For this review, take the finished solid that the model builds, in its own axes (mm). A direction names the side the tool comes from. Give positions to 0.01 mm unless a question says otherwise; leave off trailing zeros. Write each loop counter-clockwise with the first axis right and the second up, starting at its lowest first coordinate (ties: lowest second). Pieces come first, ordered by that corner, then holes. Notation, with made-up numbers: M 22,65.5 L 67,65.5 A20 cw 67,84.5 Z; hole C 19.5,37.25 d8. An arc over 180 degrees is marked long. Write item = value, one per line.
```python
from build123d import *

# Parameters (mm, degrees)
SKETCH_1_R          = 1.5
SKETCH_1_R_2        = 2.5
EXTRUDE_1_DEPTH     = 10.3
CUT_EXTRUDE_1_DEPTH = 3.8
FILLET_1_R          = 2
FILLET_2_R          = 1
FILLET_3_R          = 1
FILLET_4_R          = 1


with BuildPart() as part:
    # 草图1 → 凸台-拉伸1 (new body)
    with BuildSketch(Plane(origin=(0, 0, 0), x_dir=(1, 0, 0), z_dir=(0, 1, 0))):
        Polygon((0, 12), (0, 0), (12, 0), (12, 0.9), (18, 0.9), (18, 0), (30, 0), (30, 12), (18, 12), (18, 11.1), (12, 11.1), (12, 12), align=None)
        with Locations(Location((2.5, 3, 0), (0, 0, 90))):
            Circle(SKETCH_1_R, mode=Mode.SUBTRACT)
        with Locations(Location((15, 6, 0), (0, 0, 90))):
            Circle(SKETCH_1_R_2, mode=Mode.SUBTRACT)
        with Locations(Location((27.5, 3, 0), (0, 0, 90))):
            Circle(SKETCH_1_R, mode=Mode.SUBTRACT)
        with Locations(Location((2.5, 9, 0), (0, 0, 90))):
            Circle(SKETCH_1_R, mode=Mode.SUBTRACT)
        with Locations(Location((27.5, 9, 0), (0, 0, 90))):
            Circle(SKETCH_1_R, mode=Mode.SUBTRACT)
    extrude(amount=EXTRUDE_1_DEPTH)

    # 草图2 → 切除-拉伸1 (cut)
    with BuildSketch(Plane(origin=(0, 10.3, 0), x_dir=(1, 0, 0), z_dir=(0, 1, 0))):
        Polygon((10.265727793, 6), (12.632863896, 1.9), (17.367136104, 1.9), (19.734272207, 6), (17.367136104, 10.1), (12.632863896, 10.1), align=None)
    extrude(amount=-CUT_EXTRUDE_1_DEPTH, mode=Mode.SUBTRACT)

    # 圆角1
    fillet_1_edges = [part.edges().sort_by_distance(p)[0] for p in [
        (30, 5.15, -12),
        (30, 5.15, 0),
        (0, 5.15, 0),
        (0, 5.15, -12),
    ]]
    fillet(fillet_1_edges, radius=FILLET_1_R)

    # 圆角2
    fillet_2_edges = [part.edges().sort_by_distance(p)[0] for p in [
        (10.265727793, 8.4, -6),
        (12.632863896, 8.4, -10.1),
        (17.367136104, 8.4, -10.1),
        (19.734272207, 8.4, -6),
        (17.367136104, 8.4, -1.9),
        (12.632863896, 8.4, -1.9),
    ]]
    fillet(fillet_2_edges, radius=FILLET_2_R)

    # 圆角3
    # the kernel refuses this fillet: 1 mm, written as the material it adds along each edge
    with BuildSketch(Plane(origin=(12, 0, -0.9), x_dir=(0, 0, 1), z_dir=(0, 1, 0))) as fillet_3_piece_1:
        with BuildLine():
            CenterArc((1, 0.994987437), FILLET_3_R, 180, 84.260829523)
            Line((0, 0.994987437), (-0.02, 0.994987437))
            Line((-0.02, 0.994987437), (-0.02, 0))
            Line((-0.02, 0), (0, -0.02))
            ThreePointArc((0, -0.02), (0.45, -0.02), (0.898, -0.019899749))
            Line((0.898, -0.019899749), (0.9, 0))
        make_face()
    extrude(amount=10.3)
    with BuildSketch(Plane(origin=(18, 0, -0.9), x_dir=(-1, 0, 0), z_dir=(0, 1, 0))) as fillet_3_piece_2:
        with BuildLine():
            CenterArc((0.994987437, 1), FILLET_3_R, 185.739170477, 84.260829523)
            Line((0, 0.9), (-0.019899749, 0.898))
            ThreePointArc((-0.019899749, 0.898), (-0.02, 0.45), (-0.02, 0))
            Line((-0.02, 0), (0, -0.02))
            Line((0, -0.02), (0.994987437, -0.02))
            Line((0.994987437, -0.02), (0.994987437, 0))
        make_face()
    extrude(amount=10.3)
    with BuildSketch(Plane(origin=(12, 0, -11.1), x_dir=(0, 0, -1), z_dir=(0, 1, 0))) as fillet_3_piece_3:
        with BuildLine():
            CenterArc((1, -0.994987437), FILLET_3_R, 95.739170477, 84.260829523)
            Line((0, -0.994987437), (-0.02, -0.994987437))
            Line((-0.02, -0.994987437), (-0.02, 0))
            Line((-0.02, 0), (0, 0.02))
            ThreePointArc((0, 0.02), (0.45, 0.02), (0.898, 0.019899749))
            Line((0.898, 0.019899749), (0.9, 0))
        make_face()
    extrude(amount=10.3)
    with BuildSketch(Plane(origin=(18, 0, -11.1), x_dir=(-1, 0, 0), z_dir=(0, 1, 0))) as fillet_3_piece_4:
        with BuildLine():
            CenterArc((0.994987437, -1), FILLET_3_R, 90, 84.260829523)
            Line((0, -0.9), (-0.019899749, -0.898))
            ThreePointArc((-0.019899749, -0.898), (-0.02, -0.45), (-0.02, 0))
            Line((-0.02, 0), (0, 0.02))
            Line((0, 0.02), (0.994987437, 0.02))
            Line((0.994987437, 0.02), (0.994987437, 0))
        make_face()
    extrude(amount=10.3)

    # 圆角4
    fillet_4_edges = [part.edges().sort_by_distance(p)[0] for p in [
        (18, 5.15, 0),
        (12, 5.15, 0),
        (12, 5.15, -12),
        (18, 5.15, -12),
    ]]
    fillet(fillet_4_edges, radius=FILLET_4_R)


solid = part.part
```
1. Machinability: for faces 4 (the face through (26, 5, -9)), 5 (the face through (15, 5, -11.1)), 6 (the face through (18.56, 8.43, -8.03)), which of the approach directions +Z, -Z, +X, -X, +Y, -Y give a long, thin tool a straight path to every point of the face, cutting with its end or side? Answer none if there is none.
Responses:
face_4 = +Y, -Y
face_5 = -Z, +Y, -Y
face_6 = +Y
2. We need section A-A, the plane z = -6. Write out the cut boundary in (x, y).
Responses:
outline = M 0,0 L 12.5,0 L 12.5,6.5 L 10.42,6.5 L 10.42,10.3 L 0,10.3 Z; M 17.5,0 L 30,0 L 30,10.3 L 19.58,10.3 L 19.58,6.5 L 17.5,6.5 Z
3. We need section C-C, the plane x = 15. Write out the cut boundary in (y, z), then the cut area to 3 significant figures.
Responses:
outline = M 0,-11.1 L 10.3,-11.1 L 10.3,-10.1 L 6.5,-10.1 L 6.5,-8.5 L 0,-8.5 Z; M 0,-3.5 L 6.5,-3.5 L 6.5,-1.9 L 10.3,-1.9 L 10.3,-0.9 L 0,-0.9 Z
area = 41.4 mm2
4. We need section B-B, the plane x = 2.5. Write out the cut boundary in (y, z), then the cut area to 3 significant figures.
Responses:
outline = M 0,-12 L 10.3,-12 L 10.3,-10.5 L 0,-10.5 Z; M 0,-7.5 L 10.3,-7.5 L 10.3,-4.5 L 0,-4.5 Z; M 0,-1.5 L 10.3,-1.5 L 10.3,0 L 0,0 Z
area = 61.8 mm2
5. For line 1 along X through (y, z) = (6, -9); line 2 along Z through (x, y) = (27.5, 5); line 3 along X through (y, z) = (8.25, -3), list the stretches that pass through material, from the lowest coordinate up. Write a range as from..to.
Responses:
line_1 = 0..1, 4..26, 29..30
line_2 = -12..-10.5, -7.5..-4.5, -1.5..0
line_3 = 0..1, 4..12, 18..26, 29..30
6. We need section D-D, the plane y = 1.25. Write out the cut boundary in (x, z), then the cut area to 3 significant figures.
Responses:
outline = M 0,-10 A2 ccw 2,-12 L 11.32,-12 A1 ccw 12.16,-11.55 A1 cw 12.99,-11.1 L 17.01,-11.1 A1 cw 17.84,-11.55 A1 ccw 18.68,-12 L 28,-12 A2 ccw 30,-10 L 30,-2 A2 ccw 28,0 L 18.68,0 A1 ccw 17.84,-0.45 A1 cw 17.01,-0.9 L 12.99,-0.9 A1 cw 12.16,-0.45 A1 ccw 11.32,0 L 2,0 A2 ccw 0,-2 Z; hole C 2.5,-9 d3; hole C 2.5,-3 d3; hole C 15,-6 d5; hole C 27.5,-9 d3; hole C 27.5,-3 d3
area = 298 mm2
7. The part is to be moulded in two halves that separate along X. For faces 1 (the face through (15, 5, -0.9)), 2 (the face through (0.57, 5.22, -11.4)), 3 (the face through (23, 5, -12)), say which applies: +X half, -X half, draft (parallel to the pull), parting line (faces both ways), or undercut.
Responses:
face_1 = undercut
face_2 = -X half
face_3 = draft
8. Insertion check: P1, Ø6, axis at x = 15, z = -6, coming from the -Y side; P2, Ø1.2, axis at x = 16, y = 7.5, coming from the +Z side; P3, Ø1.1, axis at x = 15, y = 8.5, coming from the -Z side; P4, Ø2.5, axis at x = 13.5, z = -7, coming from the +Y side. Each pin has a flat end and moves straight along its axis. Give the tip position at first contact, or say it passes through.
Responses:
P1 = 0
P2 = -0.9
P3 = -11.1
P4 = 6.5
